Geometry check sheet. Reference: the model listing, model coordinates, mm. Coordinates: 2 decimals unless noted, no trailing zeros. Loops run counter-clockwise (first coordinate to the right, second up) from the corner with the lowest first, then second, coordinate; pieces in that order, holes last. Notation, with made-up numbers: (-24, -3.75) - (-19, -3.75) arc R19 ccw to (-19, 2.25) - close; hole circle Ø1 at (60.5, 1.25). An arc over 180 degrees is marked (long way). Write each question's results on one line, items separated by ' | '. Start each with the question number.
(1) Sectioned sample at A-A (x = 61). Enter the section's corners in (y, z).
(2) Go/stop test with a flat-tipped pin: pin 1 Ø1.5 at (x, y) = (74, 1) entering from +Z. Record where the tip stops, or that it passes through.
(3) Material ranges on probe 1 along Y at (x, z) = (57, -0.1); probe 2 along Z at (x, y) = (99.5, 0.25); probe 3 along Y at (x, z) = (55, -1.3), recorded low to high.
from build123d import *

# Parameters (mm, degrees)
SKETCH1_R           = 2
BOSS_EXTRUDE1_DEPTH = 105
CHAMFER1_SIZE       = 0.5
CHAMFER2_SIZE       = 0.5


with BuildPart() as part:
    # Sketch1 → Boss-Extrude1 (new body)
    with BuildSketch(Plane(origin=(0, 0, 0), x_dir=(0, 0, -1), z_dir=(1, 0, 0))):
        Circle(SKETCH1_R)
    extrude(amount=BOSS_EXTRUDE1_DEPTH)

    # Chamfer1
    chamfer1_edges = [part.edges().sort_by_distance(p)[0] for p in [
        (0, 0, 2),
    ]]
    chamfer(chamfer1_edges, length=CHAMFER1_SIZE)

    # Chamfer2
    chamfer2_edges = [part.edges().sort_by_distance(p)[0] for p in [
        (105, 0, 2),
    ]]
    chamfer(chamfer2_edges, length=CHAMFER2_SIZE)


solid = part.part
Outcome:
1) outline: circle Ø4 at (0, 0)
2) pin 1: stops at z = 1.98
3) probe 1: y = -2 to 2 | probe 2: z = -1.98 to 1.98 | probe 3: y = -1.52 to 1.52
